from build123d import *

# Parameters (mm, degrees)
F0_R      = 88.9
F3_R      = 114.3
F3_R_2    = 3.175
F4_DEPTH  = 12.7
F5_R      = 114.3
F5_R_2    = 3.4925
F6_DEPTH  = 12.7
F7_R      = 3.175
F9_R      = 25.4
F10_DEPTH = 203.2
F13_ANGLE = 135


with BuildPart() as f2:
    # F2: sweep along a path in F1
    with BuildLine(Plane.XY) as f2_path:
        ThreePointArc((-44.6369265441, -107.7640477113), (-11.6005728266, -58.3214793019), (0, 0))
    # F0 (on Front) → F2 (sweep)
    with BuildSketch(Plane.XZ):
        Circle(F0_R)
    sweep(path=f2_path.line)

    # F3 (on face) → F4 (join)
    with BuildSketch(Plane(origin=(0, 0, 0), x_dir=(-1, 0, 0), z_dir=(0, 1, 0))):
        Circle(F3_R)
        with Locations((-71.8420489686, -71.8420489686)):
            Circle(F3_R_2, mode=Mode.SUBTRACT)
        with Locations((0, -101.6)):
            Circle(F3_R_2, mode=Mode.SUBTRACT)
        with Locations((71.8420489686, -71.8420489686)):
            Circle(F3_R_2, mode=Mode.SUBTRACT)
        with Locations((-101.6, 0)):
            Circle(F3_R_2, mode=Mode.SUBTRACT)
        with Locations((-71.8420489686, 71.8420489686)):
            Circle(F3_R_2, mode=Mode.SUBTRACT)
        with Locations((101.6, 0)):
            Circle(F3_R_2, mode=Mode.SUBTRACT)
        with Locations((0, 101.6)):
            Circle(F3_R_2, mode=Mode.SUBTRACT)
        with Locations((71.8420489686, 71.8420489686)):
            Circle(F3_R_2, mode=Mode.SUBTRACT)
    extrude(amount=F4_DEPTH)

    # F5 (on face) → F6 (join)
    with BuildSketch(Plane(origin=(-76.200772477, -76.1997982148, 0), x_dir=(0.7071022608, -0.7071113015, 0), z_dir=(-0.7071113015, -0.7071022608, 0))):
        with Locations((44.6383043625, 0)):
            Circle(F5_R)
        with Locations((-27.2037446061, -71.8420489686)):
            Circle(F5_R_2, mode=Mode.SUBTRACT)
        with Locations((44.6383043625, -101.6)):
            Circle(F5_R_2, mode=Mode.SUBTRACT)
        with Locations((116.480353331, -71.8420489686)):
            Circle(F5_R_2, mode=Mode.SUBTRACT)
        with Locations((-56.9616956375, 0)):
            Circle(F5_R_2, mode=Mode.SUBTRACT)
        with Locations((-27.2037446061, 71.8420489686)):
            Circle(F5_R_2, mode=Mode.SUBTRACT)
        with Locations((44.6383043625, 101.6)):
            Circle(F5_R_2, mode=Mode.SUBTRACT)
        with Locations((146.2383043625, 0)):
            Circle(F5_R_2, mode=Mode.SUBTRACT)
        with Locations((116.480353331, 71.8420489686)):
            Circle(F5_R_2, mode=Mode.SUBTRACT)
    extrude(amount=F6_DEPTH)

    # F7
    f7_edges = [f2.edges().sort_by_distance(p)[0] for p in [
        (-125.458715, -26.941226, 0),
        (114.3, 0, 0),
    ]]
    fillet(f7_edges, radius=F7_R)


with BuildPart() as f10:
    # F9 (on Front) → F10 (new body)
    with BuildSketch(Plane.XZ):
        with Locations((-25.4, 0)):
            Circle(F9_R)
    extrude(amount=F10_DEPTH)


with BuildPart() as f10_1:
    # F11: moved
    add(f10.part.moved(Location((0, 25.4, 0))))


with BuildPart() as f2_1:
    add(f2.part)

    # F12: cut F10
    add(f10_1.part, mode=Mode.SUBTRACT)


with BuildPart() as f2_2:
    # F13: moved
    add(f2_1.part.rotate(Axis((0, 0, 85.4904651642), (0, 0, 1)), F13_ANGLE))


solid = f2_2.part
Input: part model. Units: mm. Frame: model coordinates. Round coordinates to 2 decimals unless told otherwise and drop trailing zeros.
1) Ray query, L1, parallel to X at y = 122.5, z = 72.5; L2, parallel to Z at x = 21.5, y = -19; L3, parallel to Z at x = 102.5, y = 49. Return the intervals inside material, ascending.
2) Contact query for flat-ended pins moving along their axis: P1, Ø5.5, axis at y = -27.2, z = -71.84, coming from the -X side; P2, Ø10, axis at y = -15.5, z = -84, coming from the -X side; P3, Ø12, axis at y = -24.5, z = 62, coming from the -X side; P4, Ø5.5, axis at y = 146.24, z = 0, coming from the -X side. Output: stop coordinate, or through.
3) Draft query along Y for faces 1 (the flat face through (-10.11, -7.85, 1.6)), 2 (the cylindrical face through (114.025, 118.357, 74.787)), 3 (the cylindrical face through (71.52, -82.66, 34.33)). Return one class per face: pulls with the +Y half, pulls with the -Y half, needs draft (parallel to the pull), parting line crosses it, or undercut.
Geometry says:
1. L1: x = 107.76 to 120.46
1. L2: z = -84.17 to -25.19, 25.19 to 84.17
1. L3: z = -88.79 to -22.15, 22.15 to 88.79
2. P1: stops at x = 6.49
2. P2: stops at x = -7.46
2. P3: stops at x = 0.54
2. P4: passes through
3. face 1: pulls with the -Y half
3. face 2: undercut
3. face 3: parting line crosses it
